Build history of the part. All positions in model axes, mm. A direction names the side the tool comes from. Give positions to 0.01 mm unless a question says otherwise; leave off trailing zeros. Order: outer loops, then holes, each group sorted by start corner. A loop starts at its lowest first (then second) coordinate and runs counter-clockwise, first axis right, second up. Notation, with made-up numbers: M 20.25,19 L 60.25,19 A17 cw 60.25,48 Z; hole C 65.5,48 d4. An arc over 180 degrees is marked long. Use CSV: the item, a comma, the result in double quotes. Start each with the question number.
Item 1: Band-saw the part on D-D on x = -50. Write the cut outline in (y, z).
Item 2: Band-saw the part on A-A on x = 64.5. Write the cut outline in (y, z), plus the area to 3 significant figures.
Item 3: Pin check, flat tips, straight feed: P1, Ø5, axis at x = -8, y = 32, coming from the +Z side; P2, Ø5, axis at x = 64.5, y = 34, coming from the +Z side. Stop position of each tip, or through.
Item 4: Which spindle directions (+Z, -Z, +X, -X, +Y, -Y) get a long thin tool onto all of the face, cutting with end or side? Do faces 1 (the flat face through (-97, -1, -4)), 2 (the cylindrical face through (-71.647, -33.862, -2.958)), 3 (the cylindrical face through (75, -20, -5)). Say none if no direction does.
Item 5: Band-saw the part on C-C on z = -1.5. Write the cut outline in (x, y), plus the area to 3 significant figures.
Item 6: Two-plate mould, pull along X, no slides. Class faces 4 (the flat face through (-1, 28, 0)), 5 (the cylindrical face through (62, -35.917, -2.958)), 6 (the cylindrical face through (95, 40, -5)): pulls with the +X half, pulls with the -X half, needs draft (parallel to the pull), parting line crosses it, or undercut.
Item 7: Band-saw the part on B-B on y = -34. Write the cut outline in (x, z), plus the area to 3 significant figures.
Item 8: Wall check: line 1 along Y through (x, z) = (64.5, -1.45); line 2 along Y through (x, z) = (64.5, -7.25); line 3 along Y through (x, z) = (-63, -2). Give the ranges that are in metal, low to high.
from build123d import *

# Parameters (mm, degrees)
F0_W     = 194
F0_H     = 82
F0_R     = 3.15
F0_W_2   = 154
F0_H_2   = 42
F0_R_2   = 1.75
F1_DEPTH = 9
F2_DEPTH = 6
F3_R     = 5


# Not quite as in the source:
# - a feature names something its author has since deleted; it is built from what else it names


with BuildPart() as f1:
    # F0 (on Top) → F1 (new body)
    with BuildSketch(Plane.XY):
        Rectangle(F0_W, F0_H)
        with Locations((-68.5, -34)):
            Circle(F0_R, mode=Mode.SUBTRACT)
        with Locations((64.5, -34)):
            Circle(F0_R, mode=Mode.SUBTRACT)
        with Locations((-68.5, 34)):
            Circle(F0_R, mode=Mode.SUBTRACT)
        Rectangle(F0_W_2, F0_H_2, mode=Mode.SUBTRACT)
        with Locations((64.5, 34)):
            Circle(F0_R, mode=Mode.SUBTRACT)
        with Locations((-68.5, 34)):
            Circle(F0_R)
        with Locations((-68.5, 34)):
            Circle(F0_R_2, mode=Mode.SUBTRACT)
        with Locations((-68.5, -34)):
            Circle(F0_R)
        with Locations((-68.5, -34)):
            Circle(F0_R_2, mode=Mode.SUBTRACT)
        with Locations((64.5, 34)):
            Circle(F0_R)
        with Locations((64.5, 34)):
            Circle(F0_R_2, mode=Mode.SUBTRACT)
        with Locations((64.5, -34)):
            Circle(F0_R)
        with Locations((64.5, -34)):
            Circle(F0_R_2, mode=Mode.SUBTRACT)
    extrude(amount=-F1_DEPTH)

    # F0 (on Top) → F2 (cut)
    with BuildSketch(Plane.XY):
        with Locations((-68.5, 34)):
            Circle(F0_R)
        with Locations((-68.5, 34)):
            Circle(F0_R_2, mode=Mode.SUBTRACT)
        with Locations((-68.5, -34)):
            Circle(F0_R)
        with Locations((-68.5, -34)):
            Circle(F0_R_2, mode=Mode.SUBTRACT)
        with Locations((64.5, 34)):
            Circle(F0_R)
        with Locations((64.5, 34)):
            Circle(F0_R_2, mode=Mode.SUBTRACT)
        with Locations((64.5, -34)):
            Circle(F0_R)
        with Locations((64.5, -34)):
            Circle(F0_R_2, mode=Mode.SUBTRACT)
    extrude(amount=-F2_DEPTH, mode=Mode.SUBTRACT)

    # F3
    f3_edges = [f1.edges().sort_by_distance(p)[0] for p in [
        (97, 41, -4.5),
        (-97, 41, -4.5),
        (-97, -41, -4.5),
        (97, -41, -4.5),
        (-77, 21, -4.5),
        (77, 21, -4.5),
        (77, -21, -4.5),
        (-77, -21, -4.5),
    ]]
    fillet(f3_edges, radius=F3_R)


solid = f1.part
Model answer:
1,outline,"M -41,-9 L -21,-9 L -21,0 L -41,0 Z; M 21,-9 L 41,-9 L 41,0 L 21,0 Z"
2,outline,"M -41,-9 L -35.75,-9 L -35.75,-6 L -37.15,-6 L -37.15,0 L -41,0 Z; M -32.25,-9 L -21,-9 L -21,0 L -30.85,0 L -30.85,-6 L -32.25,-6 Z; M 21,-9 L 32.25,-9 L 32.25,-6 L 30.85,-6 L 30.85,0 L 21,0 Z; M 35.75,-9 L 41,-9 L 41,0 L 37.15,0 L 37.15,-6 L 35.75,-6 Z"
2,area,"263 mm^2"
3,P1,"stops at z = 0"
3,P2,"stops at z = -6"
4,face 1,"+Z, -Z, -X, +Y, -Y"
4,face 2,"+Z"
4,face 3,"+Z, -Z"
5,outline,"M -97,-36 A5 ccw -92,-41 L 92,-41 A5 ccw 97,-36 L 97,36 A5 ccw 92,41 L -92,41 A5 ccw -97,36 Z; hole M -77,-16 A5 ccw -72,-21 L 72,-21 A5 ccw 77,-16 L 77,16 A5 ccw 72,21 L -72,21 A5 ccw -77,16 Z; hole C -68.5,-34 d6.3; hole C -68.5,34 d6.3; hole C 64.5,-34 d6.3; hole C 64.5,34 d6.3"
5,area,"9,320 mm^2"
6,face 4,"needs draft"
6,face 5,"undercut"
6,face 6,"pulls with the +X half"
7,outline,"M -97,-9 L -70.25,-9 L -70.25,-6 L -71.65,-6 L -71.65,0 L -97,0 Z; M -66.75,-9 L 62.75,-9 L 62.75,-6 L 61.35,-6 L 61.35,0 L -65.35,0 L -65.35,-6 L -66.75,-6 Z; M 66.25,-9 L 97,-9 L 97,0 L 67.65,0 L 67.65,-6 L 66.25,-6 Z"
7,area,"1,650 mm^2"
8,line 1,"y = -41 to -37.15, -30.85 to -21, 21 to 30.85, 37.15 to 41"
8,line 2,"y = -41 to -35.75, -32.25 to -21, 21 to 32.25, 35.75 to 41"
8,line 3,"y = -41 to -21, 21 to 41"
